```python
from build123d import *

# Parameters (mm, degrees)
CROQUIS1_W                                           = 209
CROQUIS1_H                                           = 165
SALIENTE_EXTRUIR1_DEPTH                              = 6
SALIENTE_EXTRUIR2_DEPTH                              = 20
CROQUIS5_W                                           = 110
CROQUIS5_H                                           = 23.048861143
SALIENTE_EXTRUIR3_DEPTH                              = 8.865038464
CROQUIS6_W                                           = 209
CROQUIS6_H                                           = 165
CROQUIS6_W_2                                         = 199
CROQUIS6_H_2                                         = 155
SALIENTE_EXTRUIR4_DEPTH                              = 84
CORTAR_EXTRUIR2_REACH                                = 359.208
CROQUIS8_W                                           = 23
CROQUIS8_H                                           = 19
CORTAR_EXTRUIR4_REACH                                = 254.595
CROQUIS10_R                                          = 1.25
CROQUIS10_W                                          = 10
CROQUIS10_H                                          = 15
CROQUIS9_R                                           = 2
CROQUIS9_W                                           = 16.35
CROQUIS9_H                                           = 18.6
CORTAR_EXTRUIR5_DEPTH                                = 10
AVELLANADO_PARA_TORNILLO_CON_CABEZA_PLAN_D           = 2.4
AVELLANADO_PARA_TORNILLO_CON_CABEZA_PLAN_CSINK_D     = 4.4
AVELLANADO_PARA_TORNILLO_CON_CABEZA_PLAN_CSINK_ANGLE = 90
REDONDEO1_R                                          = 2
REDONDEO2_R                                          = 2.5
MATRIZL2_COUNT                                       = 2
MATRIZL2_PITCH                                       = 60
MATRIZL3_COUNT                                       = 2
MATRIZL3_PITCH                                       = 60
CORTAR_EXTRUIR6_DEPTH                                = 10
REFRENTADO_PARA_TORNILLO_TAP_N_CON_CABEZ_D           = 3.4
REFRENTADO_PARA_TORNILLO_TAP_N_CON_CABEZ_DEPTH       = 8.2
REFRENTADO_PARA_TORNILLO_TAP_N_CON_CABEZ_CSINK_D     = 6.72
REFRENTADO_PARA_TORNILLO_TAP_N_CON_CABEZ_CSINK_ANGLE = 90
REFRENTADO_PARA_TORNILLO_TAP_N_CON_CABEZ_TIP         = 1.021463052
CORTAR_EXTRUIR7_REACH                                = 254.595
CROQUIS24_R                                          = 2.25
REDONDEO3_R                                          = 1


with BuildPart() as part:
    # Croquis1 → Saliente-Extruir1 (new body)
    with BuildSketch(Plane(origin=(40.752081892, -109.4, 0), x_dir=(-1, 0, 0), z_dir=(0, -1, 0))):
        with Locations((-149.8, 0)):
            Rectangle(CROQUIS1_W, CROQUIS1_H)
    extrude(amount=SALIENTE_EXTRUIR1_DEPTH)

    # Croquis3 → Saliente-Extruir2 (add)
    with BuildSketch(Plane(origin=(0, -109.4, 0), x_dir=(1, 0, 0), z_dir=(0, 1, 0))):
        Polygon((177.052081892, -55), (177.052081892, -21.5), (173.052081892, -21.5), (173.052081892, -59), (291.052081892, -59), (291.052081892, 59), (173.052081892, 59), (173.052081892, 21.5), (177.052081892, 21.5), (177.052081892, 55), (287.052081892, 55), (287.052081892, -55), align=None)
    extrude(amount=SALIENTE_EXTRUIR2_DEPTH)

    # Croquis5 → Saliente-Extruir3 (add)
    with BuildSketch(Plane(origin=(0, -109.4, 0), x_dir=(1, 0, 0), z_dir=(0, 1, 0))):
        with Locations((232.052081892, 43.475569429)):
            Rectangle(CROQUIS5_W, CROQUIS5_H)
        with Locations((232.052081892, -43.475569429)):
            Rectangle(CROQUIS5_W, CROQUIS5_H)
    extrude(amount=SALIENTE_EXTRUIR3_DEPTH)

    # Croquis6 → Saliente-Extruir4 (add)
    with BuildSketch(Plane(origin=(0, -109.4, 0), x_dir=(1, 0, 0), z_dir=(0, 1, 0))):
        with Locations((190.552081892, 0)):
            Rectangle(CROQUIS6_W, CROQUIS6_H)
        with Locations((190.552081892, 0)):
            Rectangle(CROQUIS6_W_2, CROQUIS6_H_2, mode=Mode.SUBTRACT)
    extrude(amount=SALIENTE_EXTRUIR4_DEPTH)

    # Croquis8 → Cortar-Extruir2 (cut, up to next)
    with BuildSketch(Plane(origin=(0, 0, -82.5), x_dir=(-1, 0, 0), z_dir=(0, 0, -1)), mode=Mode.PRIVATE) as cortar_extruir2_sk1:
        with Locations((-133.052081892, -96)):
            Rectangle(CROQUIS8_W, CROQUIS8_H)
    cortar_extruir2_tool1 = extrude(cortar_extruir2_sk1.sketch, amount=-CORTAR_EXTRUIR2_REACH, mode=Mode.PRIVATE) & part.part
    add(cortar_extruir2_tool1.solids().sort_by_distance((133.052082, -96, -82.5))[0], mode=Mode.SUBTRACT)

    # Croquis10 → Cortar-Extruir4 (cut, up to next)
    with BuildSketch(Plane.ZY.offset(-86.052081892), mode=Mode.PRIVATE) as cortar_extruir4_sk1:
        with Locations((0, -70.4)):
            Circle(CROQUIS10_R)
    cortar_extruir4_tool1 = extrude(cortar_extruir4_sk1.sketch, amount=-CORTAR_EXTRUIR4_REACH, mode=Mode.PRIVATE) & part.part
    # Croquis10 → Cortar-Extruir4 (cut, up to next)
    with BuildSketch(Plane.ZY.offset(-86.052081892), mode=Mode.PRIVATE) as cortar_extruir4_sk2:
        with Locations((0, -95.4)):
            Rectangle(CROQUIS10_W, CROQUIS10_H)
    cortar_extruir4_tool2 = extrude(cortar_extruir4_sk2.sketch, amount=-CORTAR_EXTRUIR4_REACH, mode=Mode.PRIVATE) & part.part
    add(cortar_extruir4_tool1.solids().sort_by_distance((86.052082, -70.4, 0))[0], mode=Mode.SUBTRACT)
    add(cortar_extruir4_tool2.solids().sort_by_distance((86.052082, -95.4, 0))[0], mode=Mode.SUBTRACT)

    # Croquis9 → Cortar-Extruir5 (cut)
    with BuildSketch(Plane(origin=(86.052081892, 0, 168.552081892), x_dir=(0, 0, -1), z_dir=(1, 0, 0))):
        with Locations((187.302081892, -70.4)):
            Circle(CROQUIS9_R)
        with Locations((211.152081892, -70.4)):
            Circle(CROQUIS9_R)
        with Locations((199.227081892, -70.4)):
            Rectangle(CROQUIS9_W, CROQUIS9_H)
    cortar_extruir5 = extrude(amount=CORTAR_EXTRUIR5_DEPTH, mode=Mode.SUBTRACT)

    # Croquis14 → Taladro de margen para 5/161 (revolve, cut)
    with BuildSketch(Plane(origin=(86.052081892, -70.4, 0), x_dir=(0, 0, 1), z_dir=(0, 1, 0))):
        Polygon((0, 0), (0, 23.733468714), (4.2164, 21.2), (4.2164, 0), align=None)
    taladro_de_margen_para_5_161 = revolve(axis=Axis((79.702081892, -70.4, 0), (1, 0, 0)), mode=Mode.SUBTRACT)

    # Avellanado para tornillo con cabeza plana de M21 (through all)
    with Locations(Plane(origin=(0, -115.4, 0), x_dir=(-1, 0, 0), z_dir=(0, -1, 0))):
        with Locations((-166.052081892, 58), (-166.052081892, 21), (-100.052081892, 21), (-100.052081892, 58)):
            CounterSinkHole(AVELLANADO_PARA_TORNILLO_CON_CABEZA_PLAN_D / 2, AVELLANADO_PARA_TORNILLO_CON_CABEZA_PLAN_CSINK_D / 2, counter_sink_angle=AVELLANADO_PARA_TORNILLO_CON_CABEZA_PLAN_CSINK_ANGLE)

    # Redondeo1
    redondeo1_edges = [part.edges().sort_by_distance(p)[0] for p in [
        (86.052081892, -70.4, 82.5),
        (295.052081892, -70.4, 82.5),
        (295.052081892, -70.4, -82.5),
        (86.052081892, -70.4, -82.5),
    ]]
    fillet(redondeo1_edges, radius=REDONDEO1_R)

    # Redondeo2
    redondeo2_edges = [part.edges().sort_by_distance(p)[0] for p in [
        (290.052081892, -67.4, -77.5),
        (91.052081892, -67.4, -77.5),
        (91.052081892, -67.4, 77.5),
        (290.052081892, -67.4, 77.5),
    ]]
    fillet(redondeo2_edges, radius=REDONDEO2_R)

    # MatrizL2: Taladro de margen para 5/161 ×2
    with Locations(*[(0, 0, -i * MATRIZL2_PITCH) for i in range(1, MATRIZL2_COUNT)]):
        add(taladro_de_margen_para_5_161, mode=Mode.SUBTRACT)

    # MatrizL3: Cortar-Extruir5 ×2
    with Locations(*[(0, 0, i * MATRIZL3_PITCH) for i in range(1, MATRIZL3_COUNT)]):
        add(cortar_extruir5, mode=Mode.SUBTRACT)

    # Croquis20 → Cortar-Extruir6 (cut)
    with BuildSketch(Plane.ZY.offset(-86.052081892)):
        with BuildLine():
            Line((51.75, -73.4), (51.75, -67.4))
            ThreePointArc((51.75, -67.4), (55.5, -63.65), (59.25, -67.4))
            Line((59.25, -67.4), (59.25, -73.4))
            ThreePointArc((59.25, -73.4), (55.5, -77.15), (51.75, -73.4))
        make_face()
    extrude(amount=-CORTAR_EXTRUIR6_DEPTH, mode=Mode.SUBTRACT)

    # Refrentado para tornillo tapón con cabeza plana de clavija de M31
    with Locations(Plane(origin=(0, -115.4, 0), x_dir=(-1, 0, 0), z_dir=(0, -1, 0))):
        with Locations((-284.302081892, 71.75), (-284.302081892, -71.75), (-96.802081892, -71.75), (-96.802081892, 71.75)):
            CounterSinkHole(REFRENTADO_PARA_TORNILLO_TAP_N_CON_CABEZ_D / 2, REFRENTADO_PARA_TORNILLO_TAP_N_CON_CABEZ_CSINK_D / 2, depth=REFRENTADO_PARA_TORNILLO_TAP_N_CON_CABEZ_DEPTH, counter_sink_angle=REFRENTADO_PARA_TORNILLO_TAP_N_CON_CABEZ_CSINK_ANGLE)
            with Locations((0, 0, -(REFRENTADO_PARA_TORNILLO_TAP_N_CON_CABEZ_DEPTH + REFRENTADO_PARA_TORNILLO_TAP_N_CON_CABEZ_TIP / 2))):  # 118° drill point
                Cone(0, REFRENTADO_PARA_TORNILLO_TAP_N_CON_CABEZ_D / 2, REFRENTADO_PARA_TORNILLO_TAP_N_CON_CABEZ_TIP, mode=Mode.SUBTRACT)

    # Croquis24 → Cortar-Extruir7 (cut, up to next)
    with BuildSketch(Plane.ZY.offset(-86.052081892), mode=Mode.PRIVATE) as cortar_extruir7_sk1:
        with Locations((-60, -83.4)):
            Circle(CROQUIS24_R)
    cortar_extruir7_tool1 = extrude(cortar_extruir7_sk1.sketch, amount=-CORTAR_EXTRUIR7_REACH, mode=Mode.PRIVATE) & part.part
    add(cortar_extruir7_tool1.solids().sort_by_distance((86.052082, -83.4, -60))[0], mode=Mode.SUBTRACT)

    # Redondeo3
    redondeo3_edges = [part.edges().sort_by_distance(p)[0] for p in [
        (88.552081892, -87.9, 5),
        (88.552081892, -102.9, 5),
        (88.552081892, -102.9, -5),
        (88.552081892, -87.9, -5),
        (88.552081892, -79.7, -38.85),
        (88.552081892, -61.1, -38.85),
        (88.552081892, -61.1, -22.5),
        (88.552081892, -79.7, -22.5),
        (88.552081892, -79.7, 21.15),
        (88.552081892, -61.1, 21.15),
        (88.552081892, -61.1, 37.5),
        (88.552081892, -79.7, 37.5),
    ]]
    fillet(redondeo3_edges, radius=REDONDEO3_R)


solid = part.part
```
Can you work these out from the model? Positions are in its coordinate system, mm. A direction names the side the tool comes from. Give positions to 0.01 mm unless a question says otherwise; leave off trailing zeros. Order: outer loops, then holes, each group sorted by start corner. A loop starts at its lowest first (then second) coordinate and runs counter-clockwise, first axis right, second up. Notation, with made-up numbers: M -20.5,-25 L 10.5,-25 A15 ccw 10.5,-10 Z; hole C 3,50 d9. An arc over 180 degrees is marked long. One line per item, written item: value.
1) Please list where these lines run through material, in increasing order: line 1 along Z through (x, y) = (267, -102.5); line 2 along Y through (x, z) = (89.1, 0); line 3 along Z through (x, y) = (197.5, -61.5).
Answer sheet:
line 1: z = -82.5 to -77.5, -59 to -31.95, 31.95 to 59, 77.5 to 82.5
line 2: y = -115.4 to -102.9, -87.9 to -74.62, -66.18 to -25.4
line 3: z = -82.5 to -77.5, 77.5 to 82.5
2) I want a section at B-B, the plane x = 217. List the corners of the cut face in (y, z) for me, plus the area to 3 significant figures.
Answer sheet:
outline: M -115.4,-82.5 L -25.4,-82.5 L -25.4,-77.5 L -109.4,-77.5 L -109.4,-59 L -89.4,-59 L -89.4,-55 L -100.53,-55 L -100.53,-31.95 L -109.4,-31.95 L -109.4,31.95 L -100.53,31.95 L -100.53,55 L -89.4,55 L -89.4,59 L -109.4,59 L -109.4,77.5 L -25.4,77.5 L -25.4,82.5 L -115.4,82.5 Z
area: 2,400 mm^2
3) I want a section at A-A, the plane y = -35. List the corners of the cut face in (x, z) for me, plus the area to 3 significant figures.
Answer sheet:
outline: M 86.05,-80.5 A2 ccw 88.05,-82.5 L 293.05,-82.5 A2 ccw 295.05,-80.5 L 295.05,80.5 A2 ccw 293.05,82.5 L 88.05,82.5 A2 ccw 86.05,80.5 Z; hole M 91.05,-75 A2.5 ccw 93.55,-77.5 L 287.55,-77.5 A2.5 ccw 290.05,-75 L 290.05,75 A2.5 ccw 287.55,77.5 L 93.55,77.5 A2.5 ccw 91.05,75 Z
area: 3,640 mm^2
4) For P1, Ø2.5, axis at x = 87.5, y = -71, coming from the -Z side; P2, Ø3, axis at x = 166.05, z = -58, coming from the -Y side; P3, Ø5, axis at y = -70.4, z = -60, coming from the -X side, each with a flat end and sliding along its axis, tell me the tip position at first contact or that it passes through.
Answer sheet:
P1: stops at z = -82.5
P2: stops at y = -114.7
P3: stops at x = 290.05
5) I want a section at C-C, the plane x = 119. List the corners of the cut face in (y, z) for me.
Answer sheet:
outline: M -115.4,-82.5 L -25.4,-82.5 L -25.4,-77.5 L -109.4,-77.5 L -109.4,77.5 L -25.4,77.5 L -25.4,82.5 L -115.4,82.5 Z
6) We'd pull the mould along Y, two halves only. Please class faces 5 (the face through (189, -71, -82.5)), 6 (the face through (88.52, -77.15, 55.58)), 7 (the face through (231, -100.535, -44)): released by +Y, released by -Y, zero draft, split by the parting line, or undercut.
Answer sheet:
face 5: zero draft
face 6: undercut
face 7: released by +Y
7) On a 3-axis mill with a long thin cutter (end or side, diameter ignored), from which of +Z, -Z, +X, -X, +Y, -Y can I reach the whole of each face in a straight line? I mean faces 1 (the face through (182, -25.4, 79)), 2 (the face through (91.052, -59, 1)), 3 (the face through (133, -105.5, -80)), 4 (the face through (88.517, -73.955, 2.267)). Say none if no direction works.
Answer sheet:
face 1: +Z, -Z, +X, -X, +Y
face 2: +Y
face 3: -Z
face 4: -X
